Geometry check sheet. Reference: drawing and pictorial views, mm from the part's lowest x, y, z. A direction names the side the tool comes from. Give positions to 0.01 mm unless a question says otherwise; leave off trailing zeros. Loops run counter-clockwise (first coordinate to the right, second up) from the corner with the lowest first, then second, coordinate; pieces in that order, holes last. Notation, with made-up numbers: (14, 27) - (32, 27) arc R28 cw to (32, 55) - close; hole circle Ø7 at (53.5, 37.5). An arc over 180 degrees is marked (long way). Answer in a Markdown table with one row per item. Add a question column.
(1) Draft check along Z on the marked faces 3, 4 and 5. Enter one of: released by +Z, released by -Z, zero draft, split by the parting line, or undercut.
(2) Sectioned sample at A-A on z = 8.26. Enter the section's corners in (x, y) (1 decimal), then the cut area to 3 significant figures.
(3) Sectioned sample at B-B on x = 35.5. Enter the section's corners in (y, z) (1 decimal).
(4) Sectioned sample at D-D on z = 33.5. Enter the section's corners in (x, y) (1 decimal).
(5) Thickness scan on L1, parallel to Z at x = 56.5, y = 8.5 (1 decimal); L2, parallel to X at y = 10, z = 19 (1 decimal); L3, parallel to Z at x = 15.5, y = 9.75 (1 decimal). Record the ranges inside material, lowest first.
(6) Set-up check for the marked faces 1 and 2: record each of +Z, -Z, +X, -X, +Y, -Y from which the full face is reachable in a straight line by a thin tool's end or side.
(7) Go/stop test with flat-tipped pins: P1, Ø4, axis at x = 8.26, z = 8.26, coming from the -Y side; P2, Ø6.5, axis at x = 51.5, z = 10, coming from the +Y side. Record where each tip stops, or that it passes through.
(8) Sectioned sample at C-C on x = 8.26. Enter the section's corners in (y, z) (1 decimal), then the cut area to 3 significant figures.
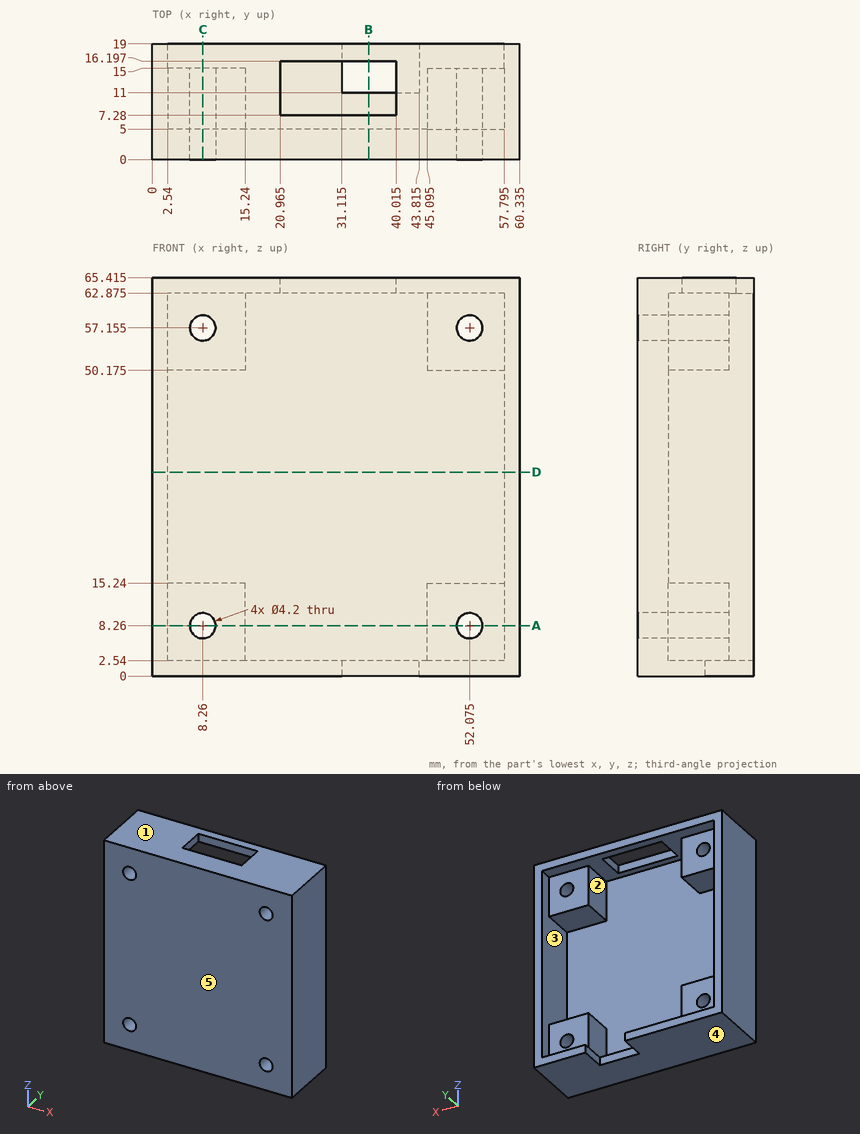
Reply:
| question | item | result |
|---|---|---|
| 1 | face 3 | undercut |
| 1 | face 4 | released by -Z |
| 1 | face 5 | zero draft |
| 2 | outline | (0, 0) - (6.2, 0) - (6.2, 15) - (2.5, 15) - (2.5, 19) - (0, 19) - close; (10.4, 0) - (50, 0) - (50, 15) - (45.1, 15) - (45.1, 5) - (15.2, 5) - (15.2, 15) - (10.4, 15) - close; (54.2, 0) - (60.3, 0) - (60.3, 19) - (57.8, 19) - (57.8, 15) - (54.2, 15) - close |
| 2 | area | 501 mm^2 |
| 3 | outline | (0, 0) - (11, 0) - (11, 2.5) - (5, 2.5) - (5, 62.9) - (7.3, 62.9) - (7.3, 65.4) - (0, 65.4) - close; (16.2, 62.9) - (19, 62.9) - (19, 65.4) - (16.2, 65.4) - close |
| 4 | outline | (0, 0) - (60.3, 0) - (60.3, 19) - (57.8, 19) - (57.8, 5) - (2.5, 5) - (2.5, 19) - (0, 19) - close |
| 5 | L1 | 0 to 15.2, 50.2 to 65.4 |
| 5 | L2 | 0 to 2.5, 57.8 to 60.3 |
| 5 | L3 | 0 to 2.5, 62.9 to 65.4 |
| 6 | face 1 | +Z, +X, -X, +Y, -Y |
| 6 | face 2 | +Y |
| 7 | P1 | through |
| 7 | P2 | y = 15 |
| 8 | outline | (0, 0) - (19, 0) - (19, 2.5) - (15, 2.5) - (15, 6.2) - (0, 6.2) - close; (0, 10.4) - (15, 10.4) - (15, 15.2) - (5, 15.2) - (5, 50.2) - (15, 50.2) - (15, 55.1) - (0, 55.1) - close; (0, 59.3) - (15, 59.3) - (15, 62.9) - (19, 62.9) - (19, 65.4) - (0, 65.4) - close |
| 8 | area | 526 mm^2 |
